Check sheet for the modelled part. Datum: model origin and axes. Units: mm. Give positions to 0.01 mm unless a question says otherwise; leave off trailing zeros. Write each loop counter-clockwise with the first axis right and the second up, starting at its lowest first coordinate (ties: lowest second). Pieces come first, ordered by that corner, then holes. Notation, with made-up numbers: (-23.75, -22) -> (-1.75, -22) arc R9 cw to (-1.75, -15) -> close; hole circle Ø2 at (77, 43). An arc over 180 degrees is marked (long way). Answer as a JSON object with one key per item and string values.
from build123d import *

# Parameters (mm, degrees)
SKETCH1_R                  = 14.2875
BOSS_EXTRUDE1_DEPTH        = 3.175
F_9_0_196_DIAMETER_HOLE1_D = 4.9784


with BuildPart() as part:
    # Sketch1 → Boss-Extrude1 (new body)
    with BuildSketch(Plane(origin=(0, 0, 0), x_dir=(0, 1, 0), z_dir=(0, 0, 1))):
        with BuildLine():
            Line((-33.655, 31.75), (0, 31.75))
            ThreePointArc((0, 31.75), (31.75, 0), (0, -31.75))
            Line((0, -31.75), (-33.655, -31.75))
            ThreePointArc((-33.655, -31.75), (-65.405, 0), (-33.655, 31.75))
        make_face()
        with Locations(Location((0, 0, 0), (0, 0, 270))):
            Circle(SKETCH1_R, mode=Mode.SUBTRACT)
        with Locations(Location((-33.655, 0, 0), (0, 0, 270))):
            Circle(SKETCH1_R, mode=Mode.SUBTRACT)
    extrude(amount=BOSS_EXTRUDE1_DEPTH)

    # #9 (0.196) Diameter Hole1 (through all)
    with Locations(Plane.XY.offset(3.175)):
        with Locations((-58.38589225, 11.773697217), (-25.4, 0), (25.4, 0), (0, -59.055), (-17.960512242, 17.960512242), (17.960512242, 17.960512242)):
            Hole(F_9_0_196_DIAMETER_HOLE1_D / 2)


solid = part.part
1. Mould release check, pull along X, two halves, no side actions. Record for faces 1 (the face through (-0.698, 31.742, 1.565)), 2 (the face through (-14.274, 0.628, 1.565)), 3 (the face through (-16.126, 19.643, 1.565)), 4 (the face through (-31.75, -17, 2)): released by +X, released by -X, zero draft, split by the parting line, or undercut.
Determined:
{"face 1": "split by the parting line", "face 2": "undercut", "face 3": "undercut", "face 4": "released by -X"}
2. Sectioned sample at B-B, the plane y = -9. Enter the section's corners in (x, z) (3 decimals).
Determined:
{"outline": "(-31.75, 0) -> (-11.097, 0) -> (-11.097, 3.175) -> (-31.75, 3.175) -> close; (11.097, 0) -> (31.75, 0) -> (31.75, 3.175) -> (11.097, 3.175) -> close"}
3. Sectioned sample at C-C, the plane x = 25. Enter the section's corners in (y, z) (3 decimals), plus the area to 3 significant figures.
Determined:
{"outline": "(-53.227, 0) -> (-2.457, 0) -> (-2.457, 3.175) -> (-53.227, 3.175) -> close; (2.457, 0) -> (19.572, 0) -> (19.572, 3.175) -> (2.457, 3.175) -> close", "area": "216 mm^2"}
4. Sectioned sample at A-A, the plane x = 0. State how many separate pieces and enclosed holes the cut face has, plus the area to 3 significant figures.
Determined:
{"separate pieces": "4", "enclosed holes": "0", "area": "111 mm^2"}
5. Scan lines: L1, parallel to Y at x = -4, z = 0.9; L2, parallel to X at y = 2, z = 1.45; L3, parallel to Y at x = -12, z = 1.4. Record each from-to range of solid material in increasing order. Write a range as [from, to].
Determined:
{"L1": "[-65.15, -47.37], [-19.94, -13.72], [13.72, 31.5]", "L2": "[-31.69, -26.88], [-23.92, -14.15], [14.15, 23.92], [26.88, 31.69]", "L3": "[-63.05, -41.41], [-25.9, -7.75], [7.75, 29.39]"}
